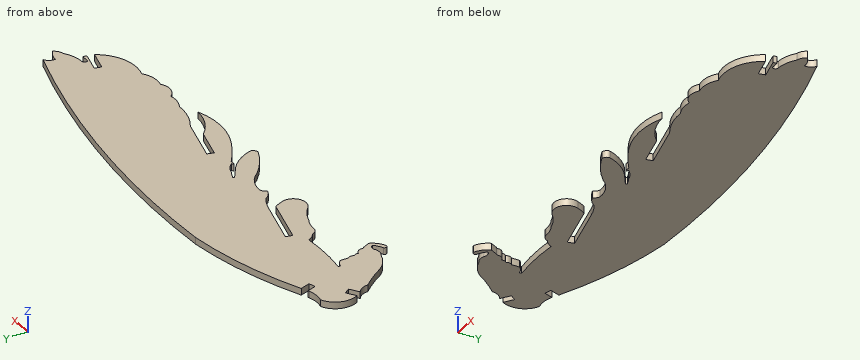
from build123d import *

# Parameters (mm, degrees)
BOSS_EXTRUDE1_DEPTH = 1.524
CUT_EXTRUDE1_DEPTH  = 1.524


with BuildPart() as part:
    # Sketch1 → Boss-Extrude1 (new body)
    with BuildSketch(Plane.XY):
        with BuildLine():
            Line((101.100291423, 60.374270727), (90.656589002, 62.891021845))
            Line((90.656589002, 62.891021845), (90.299552181, 61.409434619))
            Line((90.299552181, 61.409434619), (97.275281594, 59.728404837))
            ThreePointArc((97.275281594, 59.728404837), (100.712861052, 57.330103102), (104.811716554, 56.453640143))
            ThreePointArc((104.811716554, 56.453640143), (98.388387768, 55.183939277), (91.99420693, 56.593103707))
            ThreePointArc((91.99420693, 56.593103707), (88.820887917, 58.243640163), (85.854606826, 60.242489993))
            ThreePointArc((85.854606826, 60.242489993), (85.294961905, 60.16786255), (84.735316985, 60.242489993))
            ThreePointArc((84.735316985, 60.242489993), (84.911389048, 60.485248679), (85.199998696, 60.566720278))
            ThreePointArc((85.199998696, 60.566720278), (84.093704885, 61.559355838), (82.737345027, 62.167220368))
            ThreePointArc((82.737345027, 62.167220368), (82.242631079, 62.293353709), (81.813901616, 62.570558609))
            ThreePointArc((81.813901616, 62.570558609), (81.348307425, 62.709827468), (80.915148386, 62.930161332))
            ThreePointArc((80.915148386, 62.930161332), (80.575687035, 62.892592479), (80.689439461, 62.570558609))
            ThreePointArc((80.689439461, 62.570558609), (81.362910423, 62.034486044), (82.093679171, 61.579608074))
            ThreePointArc((82.093679171, 61.579608074), (85.34723108, 58.853595342), (87.294585764, 55.08204988))
            ThreePointArc((87.294585764, 55.08204988), (86.96715778, 54.308537604), (86.2100149, 53.944855072))
            ThreePointArc((86.2100149, 53.944855072), (82.631314085, 55.737501843), (79.510424358, 58.243640163))
            ThreePointArc((79.510424358, 58.243640163), (77.101022334, 60.220982956), (74.043252382, 60.8252557))
            ThreePointArc((74.043252382, 60.8252557), (73.319039981, 60.442919356), (72.912598281, 59.731955343))
            ThreePointArc((72.912598281, 59.731955343), (71.649210609, 60.355874406), (70.713564157, 61.409434619))
            ThreePointArc((70.713564157, 61.409434619), (69.01653018, 62.293413679), (67.185483534, 62.848941789))
            Line((67.185483534, 62.848941789), (56.741781112, 65.365692908))
            Line((56.741781112, 65.365692908), (56.384744292, 63.884105681))
            Line((56.384744292, 63.884105681), (67.187541645, 61.280818914))
            ThreePointArc((67.187541645, 61.280818914), (67.728064625, 60.371118212), (68.120097106, 59.388249456))
            ThreePointArc((68.120097106, 59.388249456), (67.25174991, 56.088088151), (63.840774779, 55.986401624))
            ThreePointArc((63.840774779, 55.986401624), (61.915192799, 57.442438875), (59.66587196, 58.319060916))
            ThreePointArc((59.66587196, 58.319060916), (58.165438165, 58.903580474), (56.56257634, 59.057848613))
            ThreePointArc((56.56257634, 59.057848613), (55.502751345, 59.425253798), (54.876523852, 60.355874406))
            ThreePointArc((54.876523852, 60.355874406), (54.009369491, 61.07018483), (53.432898123, 62.034486044))
            ThreePointArc((53.432898123, 62.034486044), (47.739513392, 61.768563203), (42.053880875, 62.167220368))
            Line((42.053880875, 62.167220368), (41.993373858, 61.698351986))
            ThreePointArc((41.993373858, 61.698351986), (42.952167328, 61.355476536), (43.743732957, 60.714951479))
            ThreePointArc((43.743732957, 60.714951479), (43.790697856, 59.811147629), (43.743732957, 58.907343779))
            ThreePointArc((43.743732957, 58.907343779), (44.082816136, 58.172570857), (43.912857263, 57.381380215))
            ThreePointArc((43.912857263, 57.381380215), (44.274457866, 56.899495102), (44.262024663, 56.297154937))
            ThreePointArc((44.262024663, 56.297154937), (45.122173078, 55.767110933), (45.378894328, 54.789923059))
            ThreePointArc((45.378894328, 54.789923059), (45.435502491, 54.514155378), (45.627787771, 54.308537604))
            Line((45.627787771, 54.308537604), (46.389355044, 52.737014998))
            ThreePointArc((46.389355044, 52.737014998), (45.400171695, 51.226760005), (43.912857263, 50.203407855))
            ThreePointArc((43.912857263, 50.203407855), (43.364944937, 50.495067499), (43.527258774, 51.094173069))
            ThreePointArc((43.527258774, 51.094173069), (44.526346213, 51.696095286), (45.400171695, 52.468698091))
            ThreePointArc((45.400171695, 52.468698091), (45.003045019, 52.919665256), (44.407834519, 53.00216035))
            ThreePointArc((44.407834519, 53.00216035), (43.983628759, 52.963097784), (43.622570614, 52.737014998))
            ThreePointArc((43.622570614, 52.737014998), (42.399406092, 52.548722507), (41.233267746, 52.963097784))
            ThreePointArc((41.233267746, 52.963097784), (38.971135138, 53.982911867), (37.161424671, 55.680619947))
            ThreePointArc((37.161424671, 55.680619947), (35.381305609, 58.306867343), (33.315602324, 60.714951479))
            ThreePointArc((33.315602324, 60.714951479), (32.966961663, 62.14091635), (31.968277944, 63.216814558))
            ThreePointArc((31.968277944, 63.216814558), (30.501031212, 67.657392256), (33.315602324, 71.392326356))
            ThreePointArc((33.315602324, 71.392326356), (35.258344298, 71.213317676), (37.161424671, 71.642940269))
            ThreePointArc((37.161424671, 71.642940269), (37.296342328, 71.710526901), (37.431371034, 71.777891398))
            Line((37.431371034, 71.777891398), (38.060215392, 69.775819105))
            Line((38.060215392, 69.775819105), (39.550898091, 70.269167956))
            Line((39.550898091, 70.269167956), (38.8265509, 72.457825788))
            ThreePointArc((38.8265509, 72.457825788), (51.785413467, 77.471627923), (65.35310261, 80.469650975))
            ThreePointArc((65.35310261, 80.469650975), (101.39539204, 79.676514857), (136.707899952, 72.416867675))
            ThreePointArc((136.707899952, 72.416867675), (135.835671661, 71.50364664), (135.569556588, 70.269167956))
            ThreePointArc((135.569556588, 70.269167956), (137.092541248, 70.02020814), (138.413889319, 69.223024009))
            ThreePointArc((138.413889319, 69.223024009), (137.71652772, 68.362597164), (136.707899952, 67.905084783))
            ThreePointArc((136.707899952, 67.905084783), (134.733670661, 66.785291795), (132.524956631, 66.262702129))
            ThreePointArc((132.524956631, 66.262702129), (131.786563313, 65.984146711), (131.909656731, 65.204617479))
            Line((131.909656731, 65.204617479), (133.736189305, 65.204617479))
            Line((133.736189305, 65.204617479), (133.535689712, 64.372609071))
            Line((133.535689712, 64.372609071), (128.90572963, 65.488349136))
            Line((128.90572963, 65.488349136), (128.54869281, 64.006761909))
            Line((128.54869281, 64.006761909), (133.178652891, 62.891021845))
            ThreePointArc((133.178652891, 62.891021845), (128.570754882, 58.881474634), (122.468796178, 58.60707916))
            ThreePointArc((122.468796178, 58.60707916), (120.00213942, 57.435104265), (117.271437866, 57.469596916))
            ThreePointArc((117.271437866, 57.469596916), (114.740756953, 56.73361331), (112.440279749, 58.01962357))
            ThreePointArc((112.440279749, 58.01962357), (110.332177288, 57.876927186), (108.32111158, 58.525057544))
            ThreePointArc((108.32111158, 58.525057544), (104.570140962, 58.900802388), (101.100291423, 60.374270727))
        make_face()
    extrude(amount=BOSS_EXTRUDE1_DEPTH)

    # Sketch2 → Cut-Extrude1 (cut)
    with BuildSketch(Plane.XY.offset(1.524)):
        Polygon((31.847119616, 63.233896416), (33.924472638, 64.695472423), (33.047527033, 65.941884236), (30.970174012, 64.480308228), align=None)
    extrude(amount=-CUT_EXTRUDE1_DEPTH, mode=Mode.SUBTRACT)


solid = part.part
Check sheet for the modelled part. Datum: model origin and axes. Units: mm. Round coordinates to 2 decimals unless told otherwise and drop trailing zeros. Write each loop counter-clockwise with the first axis right and the second up, starting at its lowest first coordinate (ties: lowest second). Pieces come first, ordered by that corner, then holes. Notation, with made-up numbers: (61, 57.5) -> (98, 57.5) arc R14 ccw to (98, 65.5) -> close; hole circle Ø10 at (2, 55). An arc over 180 degrees is marked (long way). Answer as CSV lines item,"result". Start each with the question number.
1) Material ranges on line 1 (Y direction, x = 46, z = 0.95); line 2 (Y direction, x = 79.5, z = 0.9); line 3 (Y direction, x = 66.5, z = 0.6), recorded low to high. Write a range as from..to.
2) Section check B-B on x = 121.5. Enter the section's corners in (y, z), and give its area (3 significant figures).
3) Section check A-A on x = 62. Enter the section's corners in (y, z).
4) Section check C-C on y = 76. Enter the section's corners in (x, z).
5) Go/stop test with a flat-tipped pin: P1, Ø1, axis at x = 59, y = 74, coming from the -Z side. Record where the tip stops, or that it passes through.
Found:
1,line 1,"y = 51.98..53.54, 61.82..75.51"
1,line 2,"y = 58.26..80.94"
1,line 3,"y = 55.66..61.45, 63.01..80.54"
2,outline,"(57.98, 0) -> (76.36, 0) -> (76.36, 1.52) -> (57.98, 1.52) -> close"
2,area,"28.0 mm^2"
3,outline,"(57.39, 0) -> (62.53, 0) -> (62.53, 1.52) -> (57.39, 1.52) -> close; (64.1, 0) -> (79.93, 0) -> (79.93, 1.52) -> (64.1, 1.52) -> close"
4,outline,"(47.33, 0) -> (123.13, 0) -> (123.13, 1.52) -> (47.33, 1.52) -> close"
5,P1,"stops at z = 0"
